```python
from build123d import *

# Parameters (mm, degrees)
F0_R     = 12.7
F1_DEPTH = 25.4
F2_W     = 25.4
F2_H     = 12.7
F3_DEPTH = 25.4


with BuildPart() as f1:
    # F0 (on Right) → F1 (new body)
    with BuildSketch(Plane.YZ):
        Polygon((114.3, -152.4), (114.3, 152.4), (-38.1, 152.4), (-38.1, 0), (-114.3, 0), (-114.3, -152.4), align=None)
        with Locations((76.2, -76.2)):
            Circle(F0_R, mode=Mode.SUBTRACT)
        with Locations((76.2, 76.2)):
            Circle(F0_R, mode=Mode.SUBTRACT)
    extrude(amount=F1_DEPTH)

    # F2 (on face) → F3 (cut)
    with BuildSketch(Plane(origin=(0, 0, 0), x_dir=(0, -1, 0), z_dir=(-1, 0, 0))):
        with Locations((63.5, -44.45)):
            Rectangle(F2_W, F2_H)
    extrude(amount=-F3_DEPTH, mode=Mode.SUBTRACT)


solid = f1.part
```
Can you work these out from the model? Positions are in its coordinate system, mm. A direction names the side the tool comes from. Give positions to 0.01 mm unless a question says otherwise; leave off trailing zeros. Loops run counter-clockwise (first coordinate to the right, second up) from the corner with the lowest first, then second, coordinate; pieces in that order, holes last. Notation, with made-up numbers: M -26.75,-38.75 L 21.25,-38.75 A23 ccw 21.25,-16.75 Z; hole C 2,-16 d8. An arc over 180 degrees is marked long. Use one line per item in the form item = value. Start each with the question number.
(1) I want a section at A-A, the plane x = 21. Write out the boundary of the cut face in (y, z).
(2) Please list where these lines run through material, in increasing order: line 1 (Z direction, x = 9.5, y = 76.2); line 2 (Y direction, x = 20.25, z = -42); line 3 (Z direction, x = 23.5, y = 70).
(3) On a 3-axis mill with a long thin cutter (end or side, diameter ignored), from which of +Z, -Z, +X, -X, +Y, -Y can I reach the whole of each face in a straight line? I mean faces 4 (the flat face through (13, -50.8, -45)), 5 (the flat face through (25.4, 24, 2)), 6 (the flat face through (13, -38.1, 77)). Say none if no direction works.
(4) Thinking about a two-plate mould opening in Z: for faces 1 (the flat face through (0, 24, 2)), 2 (the flat face through (13, -76, 0)), 3 (the flat face through (13, -63, -38.1)), which applies, released by +Z, released by -Z, zero draft, split by the parting line, or undercut?
(5) I want a section at D-D, the plane z = 73. Write out the boundary of the cut face in (x, y), and give its area (3 significant figures).
(6) I'm going to push flat-ended pins straight in: P1, Ø12.5, axis at x = 14.5, y = -65, coming from the +Z side; P2, Ø8, axis at x = 15, z = 76, coming from the -Y side. Where does each tip first touch, or does it pass through?
(7) I want a section at B-B, the plane z = -76.2. Write out the boundary of the cut face in (x, y), and give its area (3 significant figures).
(8) I want a section at C-C, the plane y = 76.2. Write out the boundary of the cut face in (x, z), and give its area (3 significant figures).
Worked out:
q1.outline = M -114.3,-152.4 L 114.3,-152.4 L 114.3,152.4 L -38.1,152.4 L -38.1,0 L -114.3,0 Z; hole M -76.2,-50.8 L -50.8,-50.8 L -50.8,-38.1 L -76.2,-38.1 Z; hole C 76.2,-76.2 d25.4; hole C 76.2,76.2 d25.4
q2.line_1 = -152.4 to -88.9, -63.5 to 63.5, 88.9 to 152.4
q2.line_2 = -114.3 to -76.2, -50.8 to 114.3
q2.line_3 = -152.4 to -87.28, -65.12 to 65.12, 87.28 to 152.4
q3.face_4 = +X, -X
q3.face_5 = +Z, -Z, +X, +Y, -Y
q3.face_6 = +Z, +X, -X, -Y
q4.face_1 = zero draft
q4.face_2 = released by +Z
q4.face_3 = undercut
q5.outline = M 0,-38.1 L 25.4,-38.1 L 25.4,63.91 L 0,63.91 Z; M 0,88.49 L 25.4,88.49 L 25.4,114.3 L 0,114.3 Z
q5.area = 3,250 mm²
q6.P1 = 0
q6.P2 = -38.1
q7.outline = M 0,-114.3 L 25.4,-114.3 L 25.4,63.5 L 0,63.5 Z; M 0,88.9 L 25.4,88.9 L 25.4,114.3 L 0,114.3 Z
q7.area = 5,160 mm²
q8.outline = M 0,-152.4 L 25.4,-152.4 L 25.4,-88.9 L 0,-88.9 Z; M 0,-63.5 L 25.4,-63.5 L 25.4,63.5 L 0,63.5 Z; M 0,88.9 L 25.4,88.9 L 25.4,152.4 L 0,152.4 Z
q8.area = 6,450 mm²
